Geometry check sheet. Reference: the model listing, model coordinates, mm. Face numbers are marked on the shaded views. A direction names the side the tool comes from. Coordinates: 2 decimals unless noted, no trailing zeros. Write each loop counter-clockwise with the first axis right and the second up, starting at its lowest first coordinate (ties: lowest second). Pieces come first, ordered by that corner, then holes. Notation, with made-up numbers: M -38.5,-30 L 20.5,-30 A22 cw 20.5,-4 Z; hole C 52,88 d5. An arc over 180 degrees is marked long. Answer as a JSON object with one key per item and string values. Group by question number.
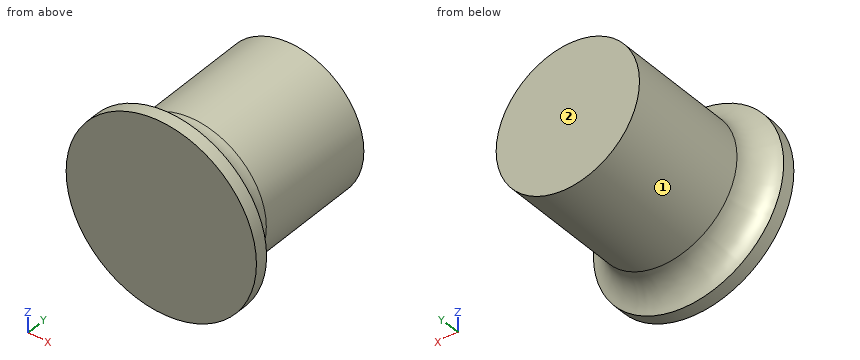
```python
from build123d import *

# Parameters (mm, degrees)
F0_R     = 11.15
F1_DEPTH = 19.3
F3_START = -1.5
F2_R     = 11.15
F2_R_2   = 8.4
F3_DEPTH = 17.8


# Not quite as in the source:
# - a fillet or chamfer that OpenCascade refuses, or shapes differently, is made with other operations: its cross-section is extruded or revolved along the edge and cut away or added


with BuildPart() as f1:
    # F0 (on Front) → F1 (new body)
    with BuildSketch(Plane.XZ):
        Circle(F0_R)
    extrude(amount=F1_DEPTH)

    # F2 (on face) → F3 (cut)
    with BuildSketch(Plane.XZ.offset(19.3).offset(F3_START)):
        Circle(F2_R)
        Circle(F2_R_2, mode=Mode.SUBTRACT)
    extrude(amount=-F3_DEPTH, mode=Mode.SUBTRACT)

    # F4: fillet of radius 3.5 on 1 edges, made by hand

    # F4_s1 → F4_t2 (revolve)
    with BuildSketch(Plane.XY):
        with BuildLine():
            ThreePointArc((11.15, -17.8), (9.1728219713, -16.5750425141), (8.4, -14.3813014172))
            Line((8.4, -14.3813014172), (8.4, -17.8))
            Line((8.4, -17.8), (11.15, -17.8))
        make_face()
    revolve(axis=Axis((0, -17.8, 0), (0, -1, 0)))


solid = f1.part
```
1) Section check B-B (z = 0). Record the cut outline in (x, y), then the cut area to 3 significant figures.
2) Go/stop test with flat-tipped pins: pin 1 Ø6 at (y, z) = (-13, -8) entering from +X; pin 2 Ø3 at (x, y) = (-2, -10.5) entering from -Z; pin 3 Ø2 at (y, z) = (-6.5, -5) entering from +X. Record where each tip stops, or that it passes through.
3) Section check C-C (y = -3.5). Record the cut outline in (x, z).
4) Material ranges on probe 1 along Z at (x, y) = (6.5, -7.75); probe 2 along Y at (x, z) = (7.5, 7.5); probe 3 along Y at (x, z) = (-9, 4), recorded low to high. Write a range as [from, to].
5) Section check A-A (x = 0). Record the cut outline in (y, z).
6) Set-up check for the marked faces 1 and 2: record each of +Z, -Z, +X, -X, +Y, -Y from which the full face is reachable in a straight line by a thin tool's end or side.
Entries:
{
 "1": {"outline": "M -11.15,-19.3 L 11.15,-19.3 L 11.15,-17.8 A3.5 cw 8.4,-14.38 L 8.4,0 L -8.4,0 L -8.4,-14.38 A3.5 cw -11.15,-17.8 Z", "area": "337 mm^2"},
 "2": {"pin 1": "x = 6.75", "pin 2": "z = -8.39", "pin 3": "x = 7.39"},
 "3": {"outline": "C 0,0 d16.8"},
 "4": {"probe 1": "[-5.32, 5.32]", "probe 2": "[-19.3, -17.63]", "probe 3": "[-19.3, -17.22]"},
 "5": {"outline": "M -19.3,-11.15 L -17.8,-11.15 A3.5 cw -14.38,-8.4 L 0,-8.4 L 0,8.4 L -14.38,8.4 A3.5 cw -17.8,11.15 L -19.3,11.15 Z"},
 "6": {"face 1": "+Y", "face 2": "+Z, -Z, +X, -X, +Y"}
}
